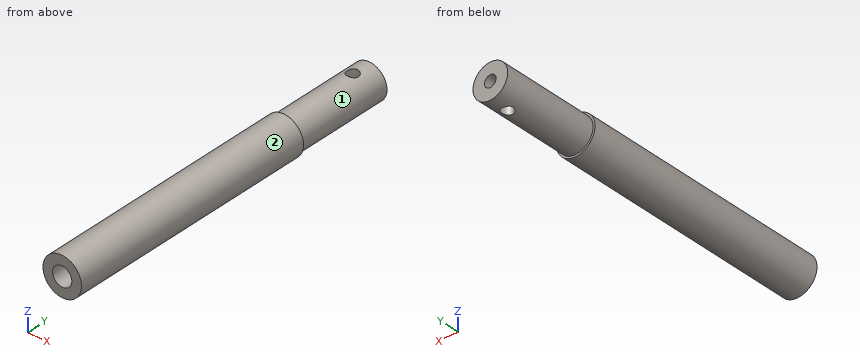
from build123d import *

# Parameters (mm, degrees)
SKETCH1_R           = 5
SKETCH1_R_2         = 2.5
BOSS_EXTRUDE1_DEPTH = 65
SKETCH2_R           = 4.5
SKETCH2_R_2         = 1.5
BOSS_EXTRUDE2_DEPTH = 25
SKETCH4_R           = 1.5
CUT_EXTRUDE1_DEPTH  = 32.5


with BuildPart() as part:
    # Sketch1 → Boss-Extrude1 (new body)
    with BuildSketch(Plane(origin=(0, 0, 0), x_dir=(1, 0, 0), z_dir=(0, 1, 0))):
        Circle(SKETCH1_R)
        Circle(SKETCH1_R_2, mode=Mode.SUBTRACT)
    extrude(amount=BOSS_EXTRUDE1_DEPTH)

    # Sketch2 → Boss-Extrude2 (add)
    with BuildSketch(Plane(origin=(0, 65, 0), x_dir=(1, 0, 0), z_dir=(0, 1, 0))):
        Circle(SKETCH2_R)
        Circle(SKETCH2_R_2, mode=Mode.SUBTRACT)
    extrude(amount=BOSS_EXTRUDE2_DEPTH)

    # Sketch4 → Cut-Extrude1 (cut, symmetric)
    with BuildSketch(Plane.XY):
        with Locations((0, 85)):
            Circle(SKETCH4_R)
    extrude(amount=CUT_EXTRUDE1_DEPTH, both=True, mode=Mode.SUBTRACT)


solid = part.part
Model file for the job. Use its own axes, mm. Face numbers are marked on the shaded views. A direction names the side the tool comes from. Give positions to 0.01 mm unless a question says otherwise; leave off trailing zeros. Order: outer loops, then holes, each group sorted by start corner. A loop starts at its lowest first (then second) coordinate and runs counter-clockwise, first axis right, second up. Notation, with made-up numbers: M 62,37.5 L 86,37.5 A22 cw 86,44.5 Z; hole C 8,21 d7. An arc over 180 degrees is marked long. Put each result on its own line as item: value. Start each with the question number.
(1) Pin check, flat tips, straight feed: pin 1 Ø1 at (x, y) = (-2.5, 19.5) entering from +Z; pin 2 Ø3 at (x, y) = (3.5, 25.5) entering from -Z; pin 3 Ø4 at (y, z) = (79, -3) entering from +X. Stop position of each tip, or through.
(2) Band-saw the part on C-C on y = 15.5. Give the cut face in (x, z).
(3) Band-saw the part on B-B on y = 82. Give the cut face in (x, z), then the cut area to 3 significant figures.
(4) Tool access for the marked faces 1 and 2: list every direction of +Z, -Z, +X, -X, +Y, -Y with a clear straight run to the whole face (end or side of a thin tool).
(5) Drill centre lines: L1, parallel to X at y = 85, z = -3.75; L2, parallel to X at y = 15, z = 0. Where is each one in solid material? Low to high. Write a range as [from, to].
(6) Band-saw the part on A-A on x = 0. Give the cut face in (y, z).
Results below:
1. pin 1: stops at z = 4.58
1. pin 2: stops at z = -4.58
1. pin 3: stops at x = 4.39
2. outline: C 0,0 d10; hole C 0,0 d5
3. outline: C 0,0 d9; hole C 0,0 d3
3. area: 56.5 mm2
4. face 1: +Y
4. face 2: +Y, -Y
5. L1: x = [-2.49, -1.5], [1.5, 2.49]
5. L2: x = [-5, -2.5], [2.5, 5]
6. outline: M 0,-5 L 65,-5 L 65,-4.5 L 83.5,-4.5 L 83.5,-1.5 L 65,-1.5 L 65,-2.5 L 0,-2.5 Z; M 0,2.5 L 65,2.5 L 65,1.5 L 83.5,1.5 L 83.5,4.5 L 65,4.5 L 65,5 L 0,5 Z; M 86.5,-4.5 L 90,-4.5 L 90,-1.5 L 86.5,-1.5 Z; M 86.5,1.5 L 90,1.5 L 90,4.5 L 86.5,4.5 Z
